Autodesk Inventor part; units mm, degrees
ref_plane "YZ Plane" through (0, 0, 0) normal (1, 0, 0) x (0, 1, 0)
ref_plane "XZ Plane" through (0, 0, 0) normal (0, 1, 0) x (-1, 0, 0)
ref_plane "XY Plane" through (0, 0, 0) normal (0, 0, 1) x (1, 0, 0)
sketch "Base" plane through (0, 0, 0) normal (0, 0, 1) x (1, 0, 0)
  line L0 (-7.25, -2.5) -> (-7.25, 2.5)
  line L1 (-7.25, 2.5) -> (-3.5, 6.25)
  line L2 (-3.5, 6.25) -> (3.5, 6.25)
  line L3 (3.5, 6.25) -> (7.25, 2.5)
  line L4 (7.25, 2.5) -> (7.25, -2.5)
  line L5 (7.25, -2.5) -> (3.5, -6.25)
  line L6 (3.5, -6.25) -> (-3.5, -6.25)
  line L7 (-3.5, -6.25) -> (-7.25, -2.5)
  line L8 (-7.25, 0) -> (7.25, 0) construction
  line L9 (0, 6.25) -> (0, -6.25) construction
  point P0 (0, 0)
  point P1 (0, 0)
  dimension "d1" = 14.5
  dimension "d5" = 12.5
  dimension "d7" = 5
extrude "BaseFeature" add sketch "Base" along normal blind 4
fillet "BaseFilletsFeature" radius 3 8 edges at (-7.25, -2.5, 2) (-3.5, -6.25, 2) (3.5, -6.25, 2) (7.25, -2.5, 2) (7.25, 2.5, 2) (3.5, 6.25, 2) (-3.5, 6.25, 2) (-7.25, 2.5, 2)
sketch "RailHoles" plane through (0, 0, 4) normal (0, 0, 1) x (1, 0, 0)
  line L0 (1.2713, 2.8219) -> (3.8219, 0.2713) construction
  line L1 (-1.7718, 0.2081) -> (0.7788, -2.3425) construction
  line L2 (6.3713, 3.3787) -> (4.3787, 5.3713) construction
  line L3 (5.375, 4.375) -> (2.5466, 1.5466) construction
  circle A0 centre (1.2713, 2.8219) radius 1
  circle A1 centre (3.8219, 0.2713) radius 1
  circle A2 centre (-1.7718, 0.2081) radius 1
  circle A3 centre (0.7788, -2.3425) radius 1
  line L4 (1.9784, 3.529) -> (4.529, 0.9784)
  line L5 (0.5642, 2.1148) -> (3.1148, -0.4358)
  line L6 (-1.0647, 0.9152) -> (1.4859, -1.6354)
  line L7 (-2.4789, -0.499) -> (0.0717, -3.0496)
  dimension "d11" = 4
  dimension "d12" = 4
  dimension "d13" = 3.6071
  dimension "d14" = 2
  dimension "d15" = 1.5
  dimension "d25" = 2.818
extrude "RailHolesFeature" cut sketch "RailHoles" against normal through all
sketch "RouteHole" plane through (-2.2574, -6.25, 0) normal (0, -1, 0) x (1, 0, 0)
  line L0 (4.5147, 4) -> (4.5147, 0) construction
  line L1 (0, 4) -> (4.5147, 4) construction
  line L2 (0, 0) -> (0, 4) construction
  line L3 (4.5147, 0) -> (0, 0) construction
  line L4 (0, 4) -> (0, 0) construction
  line L5 (0, 4) -> (4.5147, 4) construction
  line L6 (2.2574, 4) -> (2.2574, 0) construction
  line L7 (4.5147, 0) -> (0, 0) construction
  circle A0 centre (2.2574, 1.5) radius 1.25
  dimension "d40" = 2.5
  dimension "d41" = 1.5
hole "RouteHoleFeature" at (0, -6.25, 1.5) direction (0, 1, 0) diameter 2 end through all
sketch "SideProfile" plane through (7.25, -1.2574, 0) normal (1, 0, 0) x (0, 0, -1)
  arc A0 (-4, 7.5074) -> (-3, -4.9926) centre (74.625, 7.5074) ccw
  line L0 (-4, -4.9926) -> (0, -4.9926) construction
  line L1 (0, 7.5074) -> (-4, 7.5074) construction
  line L2 (-3, -4.9926) -> (0, -4.9926)
  line L3 (0, 7.5074) -> (0, -4.9926)
  line L4 (0, 7.5074) -> (0, 6.6287)
  line L5 (0, 7.5074) -> (-4, 7.5074)
  line L6 (-4, -2.1213) -> (-4, 0) construction
  dimension "d36" = 4
  dimension "d39" = 3
extrude "SideProfileFeature" cut sketch "SideProfile" against normal through all keep common part
equation "\"d7\" = 0.4 * d5"
equation "\"d12\" = 2 * d14"
equation "\"d13\" = 1.28 * d25"
properties part number "PinkyRouter"
Design review of the part built by this model. Coordinates are the model's own, in mm. A direction names the side the tool comes from. Give positions to 0.01 mm unless a question says otherwise; leave off trailing zeros. Write each loop counter-clockwise with the first axis right and the second up, starting at its lowest first coordinate (ties: lowest second). Pieces come first, ordered by that corner, then holes. Notation, with made-up numbers: M -37.5,18.5 L -26.5,18.5 A7 ccw -26.5,29.5 Z; hole C 87,28.25 d8. An arc over 180 degrees is marked long. Answer as a JSON object with one key per item and string values. Group by question number.
1) We need section B-B (x = -0.75). Count the separate pieces of the cut face and the enclosed holes in it, and give its area (3 significant figures).
2) Mouldability with a two-part tool opening along X and no side actions: class faces 3 (the face through (0, 6.25, 3)), 4 (the face through (-7.015, 2.421, 2.001)), 5 (the face through (-0.99, -4.56, 1.63)), 6 (the face through (5.36, 4.39, 1.97)) as released by +X, released by -X, zero draft, split by the parting line, or undercut.
3) Tool access review of faces 1 (the face through (7.015, -2.421, 1.846)), 2 (the face through (0.19, -0.34, 2.78)): name each direction out of +Z, -Z, +X, -X, +Y, -Y from which nothing blocks a thin tool from reaching the whole face with its end or side.
4) For line 1 along X through (y, z) = (1, 2.6); line 2 along X through (y, z) = (-3.6, 1.5); line 3 along Y through (x, z) = (-0.25, 0.5), list the stretches that pass through material, from the lowest coordinate up.
5) Clearance check with flat-ended pins moving along their axes: pin 1 Ø3 at (x, y) = (0.5, -1) entering from -Z; pin 2 Ø4 at (x, y) = (2, -4) entering from +Z; pin 3 Ø2 at (x, z) = (5, 3.5) entering from +Y. State where each tip first meets the part, or that it passes through.
6) We need section C-C (x = 5). Give the boundary of the cut face in (y, z) (3 decimals).
Answer key:
{
 "1": {"separate pieces": "4", "enclosed holes": "0", "area": "22.6 mm²"},
 "2": {"face 3": "zero draft", "face 4": "released by -X", "face 5": "undercut", "face 6": "released by +X"},
 "3": {"face 1": "+Z, -Z, +X, -Y", "face 2": "+Z, -Z"},
 "4": {"line 1": "x = -7.25 to -2.38, -1.16 to 1.68, 4.51 to 7.25", "line 2": "x = -6.15 to -1, 1 to 6.15", "line 3": "y = -6.25 to -2.73, 0.1 to 6.25"},
 "5": {"pin 1": "stops at z = 0", "pin 2": "stops at z = 3.57", "pin 3": "stops at y = 5.69"},
 "6": {"outline": "M -4.75,0 L 4.75,0 L 4.75,3.986 A78.625 ccw -4.75,3.227 Z"}
}
